Autodesk Inventor part; units mm, degrees
ref_plane "YZ Plane" through (0, 0, 0) normal (1, 0, 0) x (0, 1, 0)
ref_plane "XZ Plane" through (0, 0, 0) normal (0, 1, 0) x (-1, 0, 0)
ref_plane "XY Plane" through (0, 0, 0) normal (0, 0, 1) x (1, 0, 0)
sketch "Sketch1" plane through (0, 0, 0) normal (1, 0, 0) x (0, 1, 0)
  line L0 (2.9662, 0) -> (2.9662, -32)
  line L1 (2.9662, -32) -> (22.9662, -32)
  line L2 (22.9662, -32) -> (22.9662, -30)
  line L3 (22.9662, -30) -> (32.9662, -30)
  line L4 (32.9662, -30) -> (32.9662, -28)
  line L5 (32.9662, -28) -> (16.5117, -18.5)
  line L6 (16.5117, -18.5) -> (16.5117, -13.5)
  line L7 (16.5117, -13.5) -> (32.9662, -4)
  line L8 (32.9662, -4) -> (32.9662, -2)
  line L9 (32.9662, -2) -> (22.9662, -2)
  line L10 (22.9662, -2) -> (22.9662, 0)
  line L11 (22.9662, 0) -> (2.9662, 0)
  line L12 (0, 0) -> (34.8019, 0) construction
  line L13 (-4.5338, 0.8694) -> (-4.5338, -29.1306)
  dimension "d0" = 32
  dimension "d1" = 20
  dimension "d2" = 2
  dimension "d3" = 10
  dimension "d4" = 2
  dimension "d5" = 5
  dimension "d6" = 2
  dimension "d7" = 10
  dimension "d8" = 2
  dimension "d9" = 60
  dimension "d16" = 32.9662
  dimension "d17" = 1.8357
  dimension "d20" = 30
  dimension "d21" = 15
revolve "Revolution1" add sketch "Sketch1" angle 360 about axis through (0, -4.5338, 0.8694) along (0, 0, -1)
properties part number "Rand1"
The listing builds one solid part. Answer for the finished solid, in the listing's coordinates (mm). A direction names the side the tool comes from. Give positions to 0.01 mm unless a question says otherwise; leave off trailing zeros. Order: outer loops, then holes, each group sorted by start corner. A loop starts at its lowest first (then second) coordinate and runs counter-clockwise, first axis right, second up. Notation, with made-up numbers: (-26.5, 50) -> (31.5, 50) arc R19 ccw to (31.5, 78) -> close; hole circle Ø4 at (36, 54). An arc over 180 degrees is marked (long way). One line per item, written item: value.
1) Flat-ended cylindrical pins translate along their axes: P1, Ø5, axis at x = -27, z = -5.5, coming from the -Y side; P2, Ø5, axis at x = 4, z = -14, coming from the -Y side; P3, Ø3, axis at y = -13.5, z = -16, coming from the +X side; P4, Ø1.5, axis at y = 22.5, z = -21, coming from the +X side. Find the tip coordinate at first contact, or state that the pin passes through.
Reported:
P1: stops at y = -32.48
P2: stops at y = -28.73
P3: stops at x = 19.68
P4: passes through
2) Find section C-C, the plane z = -9.5. Determine the outline of the cut face in (x, y), plus the area to 3 significant figures.
Reported:
outline: circle Ø55.95 at (0, -4.53); hole circle Ø15 at (0, -4.53)
area: 2,280 mm^2
3) Determine the mould class of faces 1 (the cylindrical face through (0.33, -12.027, -16.224)), 2 (the conical face through (21.55, -9.319, -12.906)), 3 (the flat face through (-6, 1, -32)) for opening direction Y: pulls with the +Y half, pulls with the -Y half, needs draft (parallel to the pull), parting line crosses it, or undercut.
Reported:
face 1: undercut
face 2: parting line crosses it
face 3: needs draft
4) A tool of negligible diameter and unlimited length cuts with its end or side. For faces 4 (the flat face through (20, -24, -30)), 5 (the cylindrical face through (16.73, -26.36, -0.99)), 6 (the flat face through (-6, 1, 0)), 7 (the cylindrical face through (-6.32, 15.54, -15.96)), from which of +Z, -Z, +X, -X, +Y, -Y can it reach the whole face along a straight path? Write none if from no direction.
Reported:
face 4: -Z
face 5: +Z
face 6: +Z, +X, -X, +Y, -Y
face 7: none
5) Find section B-B, the plane z = -17. Determine the outline of the cut face in (x, y).
Reported:
outline: circle Ø42.09 at (0, -4.53); hole circle Ø15 at (0, -4.53)
6) Find section A-A, the plane x = 0. Determine the outline of the cut face in (y, z), plus the area to 3 significant figures.
Reported:
outline: (-42.03, -30) -> (-32.03, -30) -> (-32.03, -32) -> (-12.03, -32) -> (-12.03, 0) -> (-32.03, 0) -> (-32.03, -2) -> (-42.03, -2) -> (-42.03, -4) -> (-25.58, -13.5) -> (-25.58, -18.5) -> (-42.03, -28) -> close; (2.97, -32) -> (22.97, -32) -> (22.97, -30) -> (32.97, -30) -> (32.97, -28) -> (16.51, -18.5) -> (16.51, -13.5) -> (32.97, -4) -> (32.97, -2) -> (22.97, -2) -> (22.97, 0) -> (2.97, 0) -> close
area: 1,360 mm^2
7) Find the intervals of material crossed by line 1 (Z direction, x = -8, y = 30.5); line 2 (Z direction, x = -13, y = 19.5); line 3 (X direction, y = -20, z = -29.5), in increasing order.
Reported:
line 1: z = -30 to -27.1, -4.9 to -2
line 2: z = -32 to -22.13, -9.87 to 0
line 3: x = -34.16 to 34.16
